```python
from build123d import *

# Parameters (mm, degrees)
SKIZZE1_W                                           = 155.6
SKIZZE1_H                                           = 115.2
AUFSATZ_LINEAR_AUSTRAGEN1_DEPTH                     = 328.8
SCHNITT_LINEAR_AUSTRAGEN1_DEPTH                     = 328.8
SCHNITT_LINEAR_AUSTRAGEN2_DEPTH                     = 328.8
KERNLOCH_F_R_M8X1_251_D                             = 6.8
KERNLOCH_F_R_M8X1_251_DEPTH                         = 30
KERNLOCH_F_R_M8X1_251_TIP                           = 2.042926105
STIRNSENKUNG_F_R_M8_SENKSCHRAUBE_KOPF_B_D           = 9
STIRNSENKUNG_F_R_M8_SENKSCHRAUBE_KOPF_B_CBORE_D     = 22
STIRNSENKUNG_F_R_M8_SENKSCHRAUBE_KOPF_B_CBORE_DEPTH = 8
STIRNSENKUNG_F_R_M8_SENKSCHRAUBE_KO_2_D             = 9
STIRNSENKUNG_F_R_M8_SENKSCHRAUBE_KO_2_CBORE_D       = 15
STIRNSENKUNG_F_R_M8_SENKSCHRAUBE_KO_2_CBORE_DEPTH   = 8


with BuildPart() as part:
    # Skizze1 → Aufsatz-Linear austragen1 (new body)
    with BuildSketch(Plane.XY):
        Rectangle(SKIZZE1_W, SKIZZE1_H)
    extrude(amount=AUFSATZ_LINEAR_AUSTRAGEN1_DEPTH)

    # Skizze2 → Schnitt-Linear austragen1 (cut)
    with BuildSketch(Plane(origin=(77.8, 0, 0), x_dir=(0, 0, -1), z_dir=(1, 0, 0))):
        with BuildLine():
            Line((-288.8, 57.6), (-212.381166773, 57.6))
            Line((-212.381166773, 57.6), (-328.8, 118.277888245))
            Line((-328.8, 118.277888245), (-328.8, 17.6))
            ThreePointArc((-328.8, 17.6), (-317.084271247, 45.884271247), (-288.8, 57.6))
        make_face()
    schnitt_linear_austragen1 = extrude(amount=-SCHNITT_LINEAR_AUSTRAGEN1_DEPTH, mode=Mode.SUBTRACT)

    # Spiegeln1: Schnitt-Linear austragen1 across plane
    add(schnitt_linear_austragen1.mirror(Plane.ZX), mode=Mode.SUBTRACT)

    # Skizze3 → Schnitt-Linear austragen2 (cut)
    with BuildSketch(Plane(origin=(0, 57.6, 0), x_dir=(1, 0, 0), z_dir=(0, 1, 0))):
        with BuildLine():
            Line((-77.8, -328.8), (-77.8, -288.8))
            ThreePointArc((-77.8, -288.8), (-66.084271247, -317.084271247), (-37.8, -328.8))
            Line((-37.8, -328.8), (-77.8, -328.8))
        make_face()
    schnitt_linear_austragen2 = extrude(amount=-SCHNITT_LINEAR_AUSTRAGEN2_DEPTH, mode=Mode.SUBTRACT)

    # Spiegeln2: Schnitt-Linear austragen2 across plane
    add(schnitt_linear_austragen2.mirror(Plane(origin=(0, 0, 0), x_dir=(0, 0, 1), z_dir=(1, 0, 0))), mode=Mode.SUBTRACT)

    # Kernloch für M8x1.251
    with Locations(Plane(origin=(0, 0, 0), x_dir=(-1, 0, 0), z_dir=(0, 0, -1))):
        with Locations((-47.8, 0), (47.8, 0)):
            Hole(KERNLOCH_F_R_M8X1_251_D / 2, depth=KERNLOCH_F_R_M8X1_251_DEPTH)
            with Locations((0, 0, -(KERNLOCH_F_R_M8X1_251_DEPTH + KERNLOCH_F_R_M8X1_251_TIP / 2))):  # 118° drill point
                Cone(0, KERNLOCH_F_R_M8X1_251_D / 2, KERNLOCH_F_R_M8X1_251_TIP, mode=Mode.SUBTRACT)

    # Stirnsenkung f_r M8 Senkschraube _Kopf B (through all)
    with Locations(Plane(origin=(0, 57.6, 0), x_dir=(1, 0, 0), z_dir=(0, 1, 0))):
        with Locations((0, -248), (0, -60)):
            CounterBoreHole(STIRNSENKUNG_F_R_M8_SENKSCHRAUBE_KOPF_B_D / 2, STIRNSENKUNG_F_R_M8_SENKSCHRAUBE_KOPF_B_CBORE_D / 2, STIRNSENKUNG_F_R_M8_SENKSCHRAUBE_KOPF_B_CBORE_DEPTH)

    # Stirnsenkung f_r M8 Senkschraube _Ko 2 (through all)
    with Locations(Plane(origin=(0, -57.6, 0), x_dir=(-1, 0, 0), z_dir=(0, -1, 0))):
        with Locations((0, -248), (0, -60)):
            CounterBoreHole(STIRNSENKUNG_F_R_M8_SENKSCHRAUBE_KO_2_D / 2, STIRNSENKUNG_F_R_M8_SENKSCHRAUBE_KO_2_CBORE_D / 2, STIRNSENKUNG_F_R_M8_SENKSCHRAUBE_KO_2_CBORE_DEPTH)


solid = part.part
```
Build history of the part. All positions in model axes, mm. A direction names the side the tool comes from. Round coordinates to 2 decimals unless told otherwise and drop trailing zeros. Loops run counter-clockwise (first coordinate to the right, second up) from the corner with the lowest first, then second, coordinate; pieces in that order, holes last.
Item 1: Which spindle directions (+Z, -Z, +X, -X, +Y, -Y) get a long thin tool onto all of the face, cutting with end or side? Do faces 5 (the face through (-6.93, -53.66, 250.87)), 6 (the face through (0, 49.6, 65)), 7 (the face through (70.816, 0.806, 311.381)). Say none if no direction does.
Item 2: Saw through at B-B (x = 0). State how many separate pieces and enclosed holes the cut face has, then the cut area to 3 significant figures.
Item 3: Saw through at C-C (y = 23). List the corners of the cut face in (x, z).
Item 4: Drill centre lines: line 1 along Z through (x, y) = (0, 14); line 2 along X through (y, z) = (0, 19.25); line 3 along Z through (x, y) = (0, -24). Where is each one in solid material? Low to high.
Item 5: Pin check, flat tips, straight feed: P1, Ø10.5, axis at x = 0, z = 60, coming from the +Y side; P2, Ø4, axis at x = 47.8, y = 0, coming from the -Z side; P3, Ø7.5, axis at x = -3.5, z = 247.5, coming from the -Y side. Stop position of each tip, or through.
Item 6: Saw through at D-D (x = 20.5). List the corners of the cut face in (y, z), then the cut area to 3 significant figures.
Item 7: Saw through at A-A (z = 60). List the corners of the cut face in (x, y), then the cut area to 3 significant figures.
Item 8: Two-plate mould, pull along Y, no slides. Class faces 1 (the face through (1.089, -50.112, 312.102)), 2 (the face through (0.976, -53.656, 52.564)), 3 (the face through (-51.2, 0.1, 15.2)), 4 (the face through (-1, 57.6, 142)): released by +Y, released by -Y, zero draft, split by the parting line, or undercut.
Worked answers:
1. face 5: -Y
1. face 6: +Y
1. face 7: +Z, +X, +Y, -Y
2. separate pieces: 3
2. enclosed holes: 0
2. area: 34,800 mm2
3. outline: (-77.8, 0) - (77.8, 0) - (77.8, 288.8) arc R40 ccw to (43.2, 328.43) - (-43.2, 328.43) arc R40 ccw to (-77.8, 288.8) - close; hole circle Ø9 at (0, 60); hole circle Ø9 at (0, 248)
4. line 1: z = 0 to 55.5, 64.5 to 243.5, 252.5 to 328.8
4. line 2: x = -77.8 to -51.2, -44.4 to 44.4, 51.2 to 77.8
4. line 3: z = 0 to 55.5, 64.5 to 243.5, 252.5 to 328.28
5. P1: stops at y = 49.6
5. P2: stops at z = 30.84
5. P3: stops at y = -49.6
6. outline: (-57.6, 0) - (57.6, 0) - (57.6, 288.8) arc R40 ccw to (17.6, 328.8) - (-17.6, 328.8) arc R40 ccw to (-57.6, 288.8) - close
6. area: 37,200 mm2
7. outline: (-77.8, -57.6) - (-7.5, -57.6) - (-7.5, -49.6) - (-4.5, -49.6) - (-4.5, 49.6) - (-11, 49.6) - (-11, 57.6) - (-77.8, 57.6) - close; (4.5, -49.6) - (7.5, -49.6) - (7.5, -57.6) - (77.8, -57.6) - (77.8, 57.6) - (11, 57.6) - (11, 49.6) - (4.5, 49.6) - close
7. area: 16,700 mm2
8. face 1: released by -Y
8. face 2: zero draft
8. face 3: undercut
8. face 4: released by +Y
